Source: CAD feature listing. Evaluate the final solid. Frame: model axes, mm. A direction names the side the tool comes from. Coordinates: 2 decimals unless noted, no trailing zeros. Order: outer loops, then holes, each group sorted by start corner. A loop starts at its lowest first (then second) coordinate and runs counter-clockwise, first axis right, second up. Notation, with made-up numbers: (32.5, -30.75) - (51.5, -30.75) arc R30 cw to (51.5, 3.25) - close; hole circle Ø10 at (-1.75, 30). An arc over 180 degrees is marked (long way). One line per question, with ' | ' between items. Start each with the question number.
(1) Access query for faces 1 (the flat face through (-3, 40.705, 27)), 2 (the cylindrical face through (0.91, 0.53, -48.01)). Directions: +Z, -Z, +X, -X, +Y, -Y. A direction counts if a zero-diameter tool reaches every point of the face in a straight line with its end or side. Return the directions, or none.
(2) Draft query along Z for faces 3 (the flat face through (65, 0, -60)), 4 (the cylindrical face through (15.309, 63.811, -9.565)). Return one class per face: +Z half, -Z half, draft (parallel to the pull), parting line (faces both ways), or undercut.
(3) Section C-C (x = 59). Return the cut outline in (y, z), then the cut area to 3 significant figures.
(4) Section D-D (y = -60). Return the cut outline in (x, z), then the cut area to 3 significant figures.
(5) Section A-A (z = -60). Return the cut outline in (x, y).
(6) Section B-B (y = 8). Return the cut outline in (x, z), then the cut area to 3 significant figures.
(7) Line query: line 1 along X through (y, z) = (51, 35.5); line 2 along X through (y, z) = (44.5, 58.5); line 3 along Y through (x, z) = (30, -60). Output: solid intervals per line, ascending.
(8) Contact query for flat-ended pins moving along their axis: P1, Ø12, axis at y = -14.5, z = 43.5, coming from the -X side; P2, Ø10, axis at y = 48.5, z = -75, coming from the -X side; P3, Ø1, axis at x = -77.5, z = 0.5, coming from the -Y side. Output: stop coordinate, or through.
from build123d import *

# Parameters (mm, degrees)
SKETCH6_R          = 40
CUT_EXTRUDE3_DEPTH = 59.294788524860515
SKETCH13_R         = 11.999999999999975
CUT_EXTRUDE7_DEPTH = 65


with BuildPart() as part:
    # Sketch2 → Revolve2 (revolve)
    with BuildSketch(Plane.XY):
        with BuildLine():
            Line((0, 100), (2.776e-14, -100))
            ThreePointArc((2.776e-14, -100), (-100, 1.225e-14), (0, 100))
        make_face()
    revolve(axis=Axis((0, 100, 0), (1.4e-16, -1, 0)))

    # Sketch6 → Cut-Extrude3 (cut)
    with BuildSketch(Plane(origin=(-2.5379788603345292, 100, 26.23220958860291), x_dir=(-1, 0, 0), z_dir=(0, -1, 0))):
        with Locations(Location((0, 0, 0), (0, 0, 139.019257533))):
            Circle(SKETCH6_R)
    extrude(amount=CUT_EXTRUDE3_DEPTH, mode=Mode.SUBTRACT)

    # Sketch13 → Cut-Extrude7 (cut, symmetric)
    with BuildSketch(Plane(origin=(0, 0, 0), x_dir=(0, 0, -1), z_dir=(1, 0, 0))):
        with Locations((60, 0)):
            Circle(SKETCH13_R)
    extrude(amount=CUT_EXTRUDE7_DEPTH, both=True, mode=Mode.SUBTRACT)


solid = part.part
Response values:
1) face 1: +Y | face 2: none
2) face 3: undercut | face 4: undercut
3) outline: circle Ø161.48 at (0, 0); hole circle Ø24 at (0, -60) | area: 20,000 mm²
4) outline: circle Ø160 at (0, 0) | area: 20,100 mm²
5) outline: circle Ø160 at (0, 0); hole (-65, -12) - (65, -12) - (65, 12) - (-65, 12) - close
6) outline: circle Ø199.36 at (0, 0); hole (-65, -68.94) - (65, -68.94) - (65, -51.06) - (-65, -51.06) - close | area: 28,900 mm²
7) line 1: x = -78.35 to -41.45, 36.37 to 78.35 | line 2: x = -67.8 to -26.18, 21.1 to 67.8 | line 3: y = -74.16 to -12, 12 to 74.16
8) P1: stops at x = -91.72 | P2: stops at x = -53.77 | P3: stops at y = -63.8
